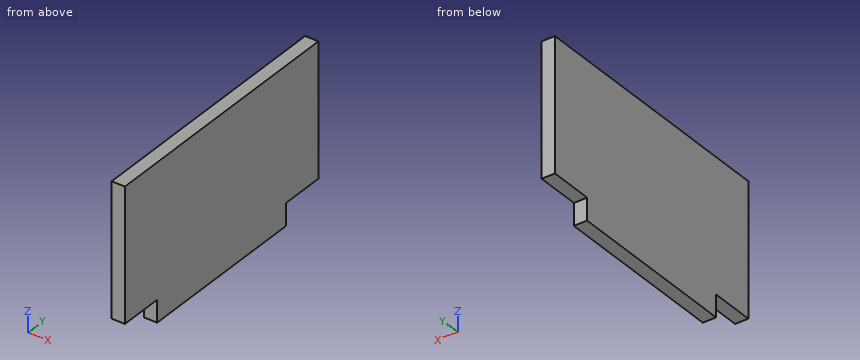
```python
from build123d import *

# Parameters (mm, degrees)
ESTRUSIONE_ESTRUSIONE1_DEPTH      = 30
ESTRUSIONE_ESTRUSIONE1_DEPTH_BACK = 5
SCHIZZO1_W                        = 3
SCHIZZO1_H                        = 40
SCHIZZO2_W                        = 3
SCHIZZO2_H                        = 30
ESTRUSIONE_ESTRUSIONE2_DEPTH      = 10


with BuildPart() as part:
    # Schizzo1 → Estrusione-Estrusione1 (new, two sides: drawn at the far end of the back side and taken through both)
    with BuildSketch(Plane.XY.offset(-ESTRUSIONE_ESTRUSIONE1_DEPTH_BACK)):
        with Locations((88.042298103, 0)):
            Rectangle(SCHIZZO1_W, SCHIZZO1_H)
    extrude(amount=ESTRUSIONE_ESTRUSIONE1_DEPTH + ESTRUSIONE_ESTRUSIONE1_DEPTH_BACK)

    # Schizzo2 → Estrusione-Estrusione2 (add)
    with BuildSketch(Plane(origin=(0, 20, 0), x_dir=(1, 0, 0), z_dir=(0, 1, 0))):
        with Locations((88.042298103, -15)):
            Rectangle(SCHIZZO2_W, SCHIZZO2_H)
    estrusione_estrusione2 = extrude(amount=ESTRUSIONE_ESTRUSIONE2_DEPTH)

    # Specchia1: Estrusione-Estrusione2 across plane
    add(estrusione_estrusione2.mirror(Plane.ZX))


solid = part.part
```
The listing builds one solid part. Answer for the finished solid, in the listing's coordinates (mm). Round coordinates to 2 decimals unless told otherwise and drop trailing zeros. Loops run counter-clockwise (first coordinate to the right, second up) from the corner with the lowest first, then second, coordinate; pieces in that order, holes last. Notation, with made-up numbers: (38, -28.75) - (79, -28.75) arc R21 cw to (79, 2.25) - close; hole circle Ø1 at (-29, 18.25). An arc over 180 degrees is marked (long way). Use one line per item in the form item = value. Start each with the question number.
1. Consider line 1 (Y direction, x = 87.15, z = -0.5); line 2 (Z direction, x = 87.4, y = 21.5). Determine where each line is inside the solid, lowest interval first. Write a range as [from, to].
2. The part is cut by section A-A on x = 89.05. Determine the outline of the cut face in (y, z), then the cut area to 3 significant figures.
3. The part is cut by section B-B on z = -3. Determine the outline of the cut face in (x, y).
4. The part is cut by section C-C on y = 25. Determine the outline of the cut face in (x, z), then the cut area to 3 significant figures.
5. Given pin 1 Ø0.9 at (x, z) = (87.5, -2) entering from -Y; pin 2 Ø1.5 at (x, y) = (88, 23) entering from -Z, each flat-ended and moving along its own axis, determine where each tip first touches the part or whether it passes through.
Geometry check:
q1.line_1 = [-20, 20]
q1.line_2 = [0, 30]
q2.outline = (-30, 0) - (-20, 0) - (-20, -5) - (20, -5) - (20, 0) - (30, 0) - (30, 30) - (-30, 30) - close
q2.area = 2,000 mm^2
q3.outline = (86.54, -20) - (89.54, -20) - (89.54, 20) - (86.54, 20) - close
q4.outline = (86.54, 0) - (89.54, 0) - (89.54, 30) - (86.54, 30) - close
q4.area = 90.0 mm^2
q5.pin_1 = -20
q5.pin_2 = 0
